Part print with two shaded views. Sizes in mm from the minimum x, y, z corner. A direction names the side the tool comes from. Round coordinates to 2 decimals unless told otherwise and drop trailing zeros. Order: outer loops, then holes, each group sorted by start corner. A loop starts at its lowest first (then second) coordinate and runs counter-clockwise, first axis right, second up. Notation, with made-up numbers: M -25,35.5 L -18,35.5 A18 cw -18,43.5 Z; hole C 28.25,-34.5 d11. An arc over 180 degrees is marked long. Answer as a JSON object with one key per item and string values.
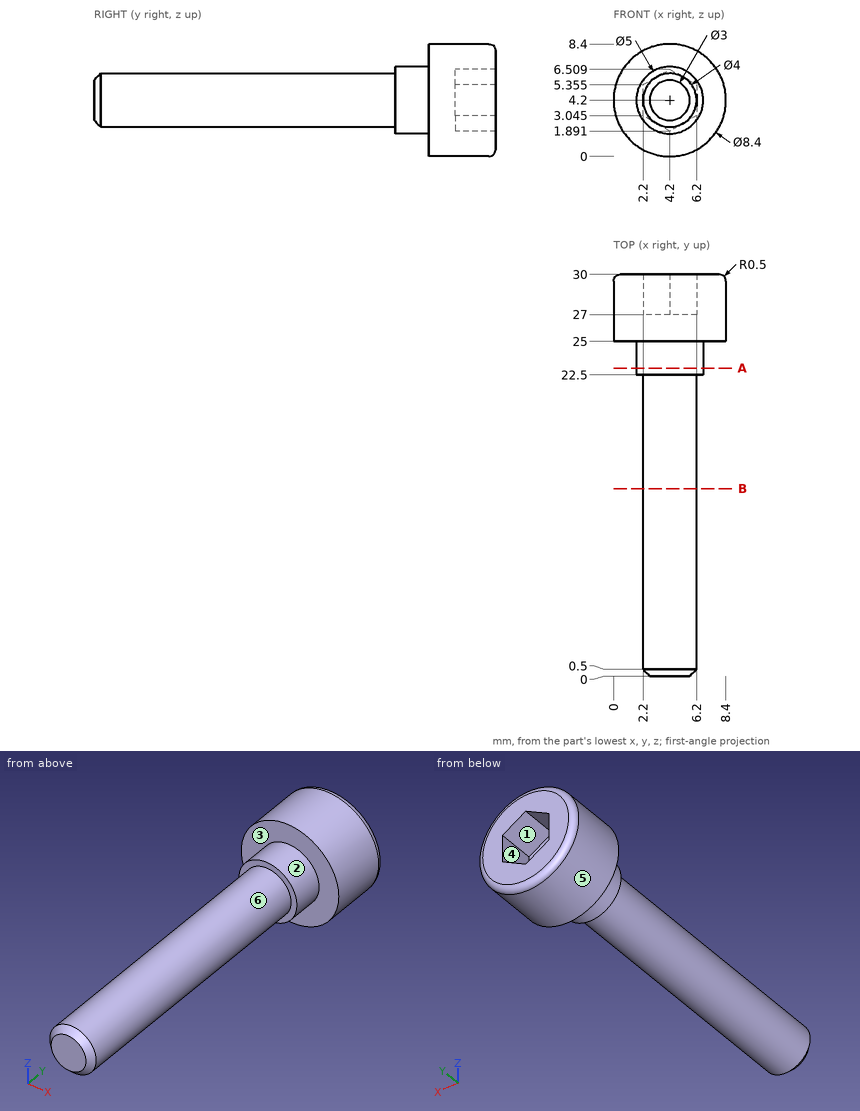
Item 1: Saw through at B-B on y = 14. List the corners of the cut face in (x, z).
Worked answers:
{"outline": "C 4.2,4.2 d4"}
Item 2: Wall check: line 1 along Z through (x, y) = (4.25, 6.5); line 2 along Y through (x, z) = (1.75, 2); line 3 along Y through (x, z) = (6, 5.75). Give the ranges that are in metal, low to high. Write a range as [from, to].
Worked answers:
{"line 1": "z = [2.2, 6.2]", "line 2": "y = [25, 30]", "line 3": "y = [22.5, 30]"}
Item 3: Saw through at A-A on y = 23. List the corners of the cut face in (x, z), and give its area (3 significant figures).
Worked answers:
{"outline": "C 4.2,4.2 d5", "area": "19.6 mm2"}
Item 4: Two-plate mould, pull along Z, no slides. Class the marked faces 1, 2, 3 and 4: released by +Z, released by -Z, zero draft, split by the parting line, or undercut.
Worked answers:
{"face 1": "undercut", "face 2": "split by the parting line", "face 3": "zero draft", "face 4": "undercut"}
Item 5: 3-axis set-ups, long thin cutter, end or side, ignore diameter. For the marked faces 5 and 6: which of +Z, -Z, +X, -X, +Y, -Y reach the whole face in a straight line?
Worked answers:
{"face 5": "+Y, -Y", "face 6": "-Y"}
Item 6: Drop flat-ended pins along their axis: pin 1 Ø2 at (y, z) = (12.5, 5.5) entering from +X; pin 2 Ø1.2 at (x, z) = (4, 4) entering from +Y; pin 3 Ø2 at (y, z) = (18.5, 7) entering from +X. Give the stop position or say it passes through.
Worked answers:
{"pin 1": "stops at x = 6.18", "pin 2": "stops at y = 27", "pin 3": "stops at x = 5.07"}
